```python
from build123d import *

# Parameters (mm, degrees)
F0_W     = 914.4
F0_H     = 1219.2
F1_DEPTH = 100.584
F2_SIZE2 = 304.8
F2_SIZE  = 76.2
F3_SIZE2 = 76.2
F3_SIZE  = 304.8


with BuildPart() as f1:
    # F0 (on Top) → F1 (new body)
    with BuildSketch(Plane.XY):
        with Locations((-2964.017556, 609.6)):
            Rectangle(F0_W, F0_H)
    extrude(amount=F1_DEPTH)

    # F2
    f2_edges = [f1.edges().sort_by_distance(p)[0] for p in [
        (-3421.217556, 609.6, 100.584),
    ]]
    chamfer(f2_edges, length=F2_SIZE, length2=F2_SIZE2)

    # F3
    f3_edges = [f1.edges().sort_by_distance(p)[0] for p in [
        (-2506.817556, 609.6, 100.584),
    ]]
    chamfer(f3_edges, length=F3_SIZE, length2=F3_SIZE2)


solid = f1.part
```
Check sheet for the modelled part. Datum: model origin and axes. Units: mm. Round coordinates to 2 decimals unless told otherwise and drop trailing zeros. Loops run counter-clockwise (first coordinate to the right, second up) from the corner with the lowest first, then second, coordinate; pieces in that order, holes last. Notation, with made-up numbers: (-24.5, -34.5) - (31.5, -34.5) arc R20 ccw to (31.5, -9.5) - close; hole circle Ø1 at (76.5, 86.5). An arc over 180 degrees is marked (long way). Answer as a JSON object with one key per item and string values. Group by question number.
Q1. Sectioned sample at A-A, the plane y = 958. Enter the section's corners in (x, z), plus the area to 3 significant figures.
Q2. Gauge pin test, flat ends, axial feed: P1, Ø5, axis at x = -3221, y = 856, coming from the +Z side; P2, Ø5, axis at x = -3009, y = 760.5, coming from the -Z side. Record the tip position at first contact, or that the pin passes through.
Q3. Sectioned sample at C-C, the plane z = 85. Enter the section's corners in (x, y), plus the area to 3 significant figures.
Q4. Scan lines: line 1 along Z through (x, y) = (-3379.5, 1129.5); line 2 along Z through (x, y) = (-3174.5, 253). Record each from-to range of solid material in increasing order. Write a range as [from, to].
Q5. Sectioned sample at B-B, the plane x = -3271. Enter the section's corners in (y, z).
Solution:
{
 "1": {"outline": "(-3421.22, 0) - (-2506.82, 0) - (-2506.82, 24.38) - (-2811.62, 100.58) - (-3116.42, 100.58) - (-3421.22, 24.38) - close", "area": "68,700 mm²"},
 "2": {"P1": "stops at z = 75.06", "P2": "stops at z = 0"},
 "3": {"outline": "(-3178.75, 0) - (-2749.28, 0) - (-2749.28, 1219.2) - (-3178.75, 1219.2) - close", "area": "524,000 mm²"},
 "4": {"line 1": "z = [0, 34.81]", "line 2": "z = [0, 86.06]"},
 "5": {"outline": "(0, 0) - (1219.2, 0) - (1219.2, 61.94) - (0, 61.94) - close"}
}
